Check sheet for the modelled part. Datum: model origin and axes. Units: mm. A direction names the side the tool comes from. Coordinates: 2 decimals unless noted, no trailing zeros. Write each loop counter-clockwise with the first axis right and the second up, starting at its lowest first coordinate (ties: lowest second). Pieces come first, ordered by that corner, then holes. Notation, with made-up numbers: (34.25, 79.5) - (57.25, 79.5) arc R22 ccw to (57.25, 95.5) - close; hole circle Ø9 at (7, -21.75). An arc over 180 degrees is marked (long way). Use one line per item in the form item = value. Start each with the question number.
1. Tool access check on faces 1 (the face through (-3, -3, 6)), 2 (the face through (-3, 3, 6)), 3 (the face through (-0.1, -4.3, 0)). Record the directions out of +Z, -Z, +X, -X, +Y, -Y that give a thin tool (end or side, any length) a straight path to the whole face; none if there is none.
2. Cross-section at B-B on z = 27.5. Record the boundary of the cut face in (x, y).
3. Cross-section at A-A on y = 2. Record the boundary of the cut face in (x, z), then the cut area to 3 significant figures.
4. Scan lines: line 1 along Y through (x, z) = (-0.25, 14); line 2 along Z through (x, y) = (2, -7); line 3 along X through (y, z) = (0.5, 8). Record each from-to range of solid material in increasing order.
5. Go/stop test with flat-tipped pins: pin 1 Ø3 at (x, z) = (5, 13.5) entering from -Y; pin 2 Ø12 at (x, z) = (-7, 24) entering from +Y; pin 3 Ø6.5 at (x, z) = (0.5, 4) entering from +Y. Record where each tip stops, or that it passes through.
6. Cross-section at D-D on y = 8.5. Record the boundary of the cut face in (x, z).
```python
from build123d import *

# Parameters (mm, degrees)
SKETCH_R     = 4
PAD_DEPTH    = 30
SKETCH001_W  = 8
SKETCH001_H  = 8
PAD001_DEPTH = 6
SKETCH002_R  = 10
PAD002_DEPTH = 10
FILLET_R     = 1


with BuildPart() as body001:
    # Sphere → Sphere (revolve)
    with BuildSketch(Plane.XZ):
        with BuildLine():
            ThreePointArc((0, -30), (30, 0), (0, 30))
            Line((0, 30), (0, -30))
        make_face()
    revolve(axis=Axis((0, 0, 0), (0, 0, 1)))


with BuildPart() as body001_1:
    # Body001 placement: moved
    add(body001.part.moved(Location((0, 0, 26))))


with BuildPart() as fillet_body:
    # Sketch → Pad (new body)
    with BuildSketch(Plane.XY):
        Circle(SKETCH_R)
    extrude(amount=PAD_DEPTH)

    # Sketch001 → Pad001 (join)
    with BuildSketch(Plane.XY):
        Rectangle(SKETCH001_W, SKETCH001_H)
    extrude(amount=PAD001_DEPTH)

    # Sketch002 → Pad002 (join)
    with BuildSketch(Plane.XY):
        Circle(SKETCH002_R)
    extrude(amount=-PAD002_DEPTH)

    # Common: intersect Body001
    add(body001_1.part, mode=Mode.INTERSECT)

    # Fillet
    fillet_edges = [fillet_body.edges().sort_by_distance(p)[0] for p in [
        (4, 4, 3),
        (-4, 4, 3),
        (-4, -4, 3),
        (4, -4, 3),
    ]]
    fillet(fillet_edges, radius=FILLET_R)


solid = fillet_body.part
```
Final values:
q1.face_1 = +Z, -X, -Y
q1.face_2 = +Z, -X, +Y
q1.face_3 = +Z
q2.outline = circle Ø8 at (0, 0)
q3.outline = (-9.8, -2.28) arc R29.93 ccw to (9.8, -2.28) - (9.8, 0) - (4, 0) - (4, 6) - (3.46, 6) - (3.46, 30) - (-3.46, 30) - (-3.46, 6) - (-4, 6) - (-4, 0) - (-9.8, 0) - close
q3.area = 281 mm²
q4.line_1 = -3.99 to 3.99
q4.line_2 = -3.1 to 0
q4.line_3 = -3.97 to 3.97
q5.pin_1 = -1.94
q5.pin_2 = 3.87
q5.pin_3 = 4
q6.outline = (-5.27, -2.28) arc R28.77 ccw to (5.27, -2.28) - (5.27, 0) - (-5.27, 0) - close
